from build123d import *

# Parameters (mm, degrees)
SKETCH_1_W              = 10
SKETCH_1_H              = 139.5
HOLE_WIZARD_6_5_6_5_1_D = 6.5
CHAMFER_1_SIZE          = 1


with BuildPart() as part:
    # 草图1 → 旋转1 (revolve)
    with BuildSketch(Plane.XY):
        with Locations((5, -60.25)):
            Rectangle(SKETCH_1_W, SKETCH_1_H)
    revolve(axis=Axis((0, 9.5, 0), (0, -1, 0)))

    # Ø6.5 (6.5) 直径孔1 (through all)
    with Locations(Plane(origin=(-10, 0, 0), x_dir=(0, 0, -1), z_dir=(-1, 0, 0))):
        with Locations((0, 0)):
            Hole(HOLE_WIZARD_6_5_6_5_1_D / 2)

    # 倒角1
    chamfer_1_edges = [part.edges().sort_by_distance(p)[0] for p in [
        (-10, 9.5, 0),
    ]]
    chamfer(chamfer_1_edges, length=CHAMFER_1_SIZE)


solid = part.part
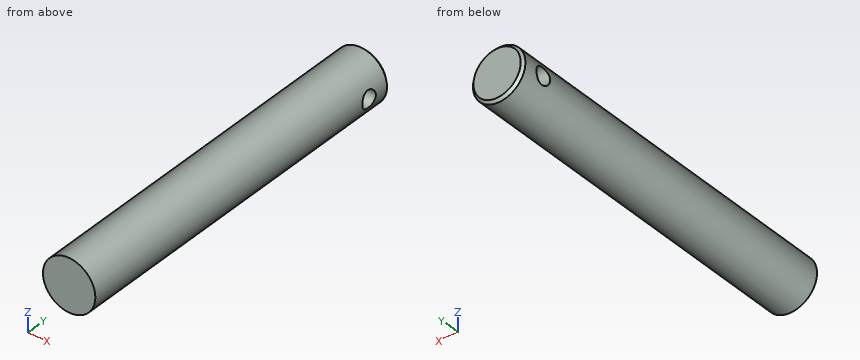
Geometry check sheet. Reference: the model listing, model coordinates, mm. Round coordinates to 2 decimals unless told otherwise and drop trailing zeros. Loops run counter-clockwise (first coordinate to the right, second up) from the corner with the lowest first, then second, coordinate; pieces in that order, holes last. Notation, with made-up numbers: (20.25, 12.25) - (72.25, 12.25) arc R13 ccw to (72.25, 27.25) - close; hole circle Ø7 at (-13, 50). An arc over 180 degrees is marked (long way). Answer as CSV lines item,"result".
(1) Material ranges on line 1 along Y through (x, z) = (4, 0); line 2 along Y through (x, z) = (-1.5, 2); line 3 along X through (y, z) = (-57, 3.25), recorded low to high.
Output values:
line 1,"y = -130 to -3.25, 3.25 to 9.5"
line 2,"y = -130 to -2.56, 2.56 to 9.5"
line 3,"x = -9.46 to 9.46"
(2) Depth check by flat-ended pin: pin 1 Ø2 at (y, z) = (-102, 8) entering from +X; pin 2 Ø5 at (y, z) = (-9.5, 7.5) entering from +X; pin 3 Ø1 at (y, z) = (-87.5, -3) entering from -X. Enter the tip coordinate at first touch or a pass-through.
Output values:
pin 1,"stops at x = 7.14"
pin 2,"stops at x = 8.66"
pin 3,"stops at x = -9.68"
(3) Cross-section at C-C, the plane y = 0. Enter the section's corners in (x, z), and give its area (3 significant figures).
Output values:
outline,"(-9.46, -3.25) arc R10 ccw to (9.46, -3.25) - close; (-9.46, 3.25) - (9.46, 3.25) arc R10 ccw to start"
area,"186 mm²"
(4) Cross-section at A-A, the plane z = 0. Enter the section's corners in (x, y), and give its area (3 significant figures).
Output values:
outline,"(-10, -130) - (10, -130) - (10, -3.25) - (-10, -3.25) - close; (-10, 3.25) - (10, 3.25) - (10, 8.5) - (9, 9.5) - (-9, 9.5) - (-10, 8.5) - close"
area,"2,660 mm²"
(5) Cross-section at B-B, the plane y = -96.5. Enter the section's corners in (x, z).
Output values:
outline,"circle Ø20 at (0, 0)"
